from build123d import *

# Parameters (mm, degrees)
F1_DEPTH  = 8
F2_R      = 1.75
F3_DEPTH  = 4.2837432044
F4_R      = 1.75
F5_DEPTH  = 25
F6_R      = 8.15
F7_DEPTH  = 2
F8_R      = 6.1
F9_DEPTH  = 5.6
F10_R     = 8.15
F11_DEPTH = 25


with BuildPart() as f1:
    # F0 (on Top) → F1 (new body)
    with BuildSketch(Plane.XY):
        with BuildLine():
            Line((18.5, 4.2827432044), (11.2097328534, 4.2827432044))
            ThreePointArc((11.2097328534, 4.2827432044), (0.2159454588, 11.9980568243), (-11.0483577501, 4.6833525412))
            Line((-11.0483577501, 4.6833525412), (-18.5, 4.6833525412))
            Line((-18.5, 4.6833525412), (-18.5, 0))
            Line((-18.5, 0), (-12, 0))
            Line((-12, 0), (12, 0))
            Line((12, 0), (18.5, 0))
            Line((18.5, 0), (18.5, 4.2827432044))
        make_face()
    extrude(amount=F1_DEPTH)

    # F2 (on face) → F3 (cut, through all)
    with BuildSketch(Plane(origin=(0, 4.2827432044, 0), x_dir=(-1, 0, 0), z_dir=(0, 1, 0))):
        with Locations((-14.5, 4)):
            Circle(F2_R)
        with Locations((14.5, 4)):
            Circle(F2_R)
    extrude(amount=-F3_DEPTH, mode=Mode.SUBTRACT)

    # F4 (on face) → F5 (cut)
    with BuildSketch(Plane(origin=(0, 4.6833525412, 0), x_dir=(-1, 0, 0), z_dir=(0, 1, 0))):
        with Locations((14.5, 4)):
            Circle(F4_R)
    extrude(amount=-F5_DEPTH, mode=Mode.SUBTRACT)

    # F6 (on face) → F7 (cut)
    with BuildSketch(Plane.XY.offset(8)):
        Circle(F6_R)
    extrude(amount=-F7_DEPTH, mode=Mode.SUBTRACT)

    # F8 (on face) → F9 (cut)
    with BuildSketch(Plane.XY.offset(6)):
        Circle(F8_R)
    extrude(amount=-F9_DEPTH, mode=Mode.SUBTRACT)

    # F10 (on face) → F11 (cut)
    with BuildSketch(Plane.XY.offset(0.4)):
        Circle(F10_R)
    extrude(amount=-F11_DEPTH, mode=Mode.SUBTRACT)


solid = f1.part
Could you check a few things on this model? Use its own coordinates, in mm. A direction names the side the tool comes from. Coordinates: 2 decimals unless noted, no trailing zeros. Order: outer loops, then holes, each group sorted by start corner. A loop starts at its lowest first (then second) coordinate and runs counter-clockwise, first axis right, second up. Notation, with made-up numbers: (49, -14) -> (68, -14) arc R11 cw to (68, 0) -> close; hole circle Ø1 at (-17.75, 76.5). An arc over 180 degrees is marked (long way). One line per item, written item: value. Start each with the question number.
1) Imagine slicing it at D-D on z = 1. List the corners of the cut face in (x, y) for me.
2) If I drill on L1, parallel to Z at x = -14.5, y = 2.95; L2, parallel to X at y = 3, z = 4.5; L3, parallel to Z at x = 6, y = 3, over which ranges is the centre line in solid material (lowest first)? Write a range as [from, to].
3) We'd pull the mould along Z, two halves only. Please class faces 4 (the cylindrical face through (-15.31, 2.37, 2.45)), 5 (the cylindrical face through (0.1, 6.1, 3.2)), 6 (the flat face through (0, 7, 6)): +Z half, -Z half, draft (parallel to the pull), parting line (faces both ways), or undercut.
4) Imagine slicing it at A-A on y = 3.75. List the corners of the cut face in (x, z) for me.
5) Which directions (+Z, -Z, +X, -X, +Y, -Y) give clear straight access to the entire face, cutting with the end or side of a thin tool? Please do faces 1 (the cylindrical face through (0.18, 8.15, 0.2)), 2 (the flat face through (17, 4.283, 4)), 3 (the flat face through (-16.4, 4.683, 3.9)).
6) I'm going to push flat-ended pins straight in: pin 1 (6.5 mm diameter, centred on x = 1, y = 3, fed in from +Z); pin 2 (1.5 mm diameter, centred on y = 5.5, z = 3, fed in from +X); pin 3 (4 mm diameter, centred on x = -9.5, z = 3.5, fed in from +Y). Where does each tip first touch, or does it pass through?
7) Imagine slicing it at C-C on z = 4. List the corners of the cut face in (x, y) for me.
8) Imagine slicing it at B-B on x = 14.5. List the corners of the cut face in (y, z) for me, plus the area to 3 significant figures.
Answer list:
1. outline: (-18.5, 0) -> (-6.1, 0) arc R6.1 cw to (6.1, 0) -> (18.5, 0) -> (18.5, 4.28) -> (11.21, 4.28) arc R12 ccw to (-11.05, 4.68) -> (-18.5, 4.68) -> close
2. L1: z = [0, 2.25], [5.75, 8]
2. L2: x = [-18.5, -16.18], [-12.82, -5.31], [5.31, 12.82], [16.18, 18.5]
2. L3: z = [0.4, 6]
3. face 4: undercut
3. face 5: draft
3. face 6: +Z half
4. outline: (-18.5, 0) -> (-7.24, 0) -> (-7.24, 0.4) -> (-4.81, 0.4) -> (-4.81, 6) -> (-7.24, 6) -> (-7.24, 8) -> (-18.5, 8) -> close; (4.81, 0.4) -> (7.24, 0.4) -> (7.24, 0) -> (18.5, 0) -> (18.5, 8) -> (7.24, 8) -> (7.24, 6) -> (4.81, 6) -> close; hole circle Ø3.5 at (-14.5, 4); hole circle Ø3.5 at (14.5, 4)
5. face 1: -Z, -Y
5. face 2: +Z, -Z, +X, +Y
5. face 3: +Z, -Z, -X, +Y
6. pin 1: stops at z = 6
6. pin 2: stops at x = 11.02
6. pin 3: stops at y = 9.37
7. outline: (-18.5, 0) -> (-16.25, 0) -> (-16.25, 4.68) -> (-18.5, 4.68) -> close; (-12.75, 0) -> (-6.1, 0) arc R6.1 cw to (6.1, 0) -> (12.75, 0) -> (12.75, 4.28) -> (11.21, 4.28) arc R12 ccw to (-11.05, 4.68) -> (-12.75, 4.68) -> close; (16.25, 0) -> (18.5, 0) -> (18.5, 4.28) -> (16.25, 4.28) -> close
8. outline: (0, 0) -> (4.28, 0) -> (4.28, 2.25) -> (0, 2.25) -> close; (0, 5.75) -> (4.28, 5.75) -> (4.28, 8) -> (0, 8) -> close
8. area: 19.3 mm2
